from build123d import *

# Parameters (mm, degrees)
F3_D     = 2.5
F3_DEPTH = 16.521
F4_SIZE  = 0.5


with BuildPart() as f1:
    # F0 (on Front) → F1 (revolve)
    with BuildSketch(Plane.XZ):
        Polygon((10, 16), (10, 0), (16.52, 0), (16.52, 2), (13.28, 11), (13.28, 15.774938604), (13.28, 16), align=None)
    revolve(axis=Axis((0, 0, 22.1384353936), (0, 0, 1)))

    # F3 (through all, one way)
    with BuildSketch(Plane.XZ):
        with Locations((0, 13.5)):
            Circle(F3_D / 2)
    extrude(amount=-F3_DEPTH, mode=Mode.SUBTRACT)

    # F4
    f4_edges = [f1.edges().sort_by_distance(p)[0] for p in [
        (-13.28, 0, 16),
        (-10, 0, 16),
        (-10, 0, 0),
        (-16.52, 0, 0),
    ]]
    chamfer(f4_edges, length=F4_SIZE)


solid = f1.part
Geometry: final body of the model. Coordinates: model frame, mm. Round coordinates to 2 decimals unless told otherwise and drop trailing zeros. Write each loop counter-clockwise with the first axis right and the second up, starting at its lowest first coordinate (ties: lowest second). Pieces come first, ordered by that corner, then holes. Notation, with made-up numbers: M 13.25,61 L 39.25,61 A19 ccw 39.25,67 Z; hole C -11,46 d6. An arc over 180 degrees is marked long. Write item = value, one per line.
Item 1: Section query A-A on x = 0. Return loops of the section in (y, z), then the cut area to 3 significant figures.
Findings:
outline = M -16.52,0.5 L -16.02,0 L -10.5,0 L -10,0.5 L -10,15.5 L -10.5,16 L -12.78,16 L -13.28,15.5 L -13.28,11 L -16.52,2 Z; M 10,0.5 L 10.5,0 L 16.02,0 L 16.52,0.5 L 16.52,2 L 13.28,11 L 13.28,12.25 L 10,12.25 Z; M 10,14.75 L 13.28,14.75 L 13.28,15.5 L 12.78,16 L 10.5,16 L 10,15.5 Z
area = 138 mm^2
Item 2: Section query D-D on z = 13.5. Return loops of the section in (x, y), then the cut area to 3 significant figures.
Findings:
outline = M -1.25,9.92 L -1.25,13.22 A13.28 ccw long 1.25,13.22 L 1.25,9.92 A10 cw long Z
area = 232 mm^2
Item 3: Pin query (flat end, axial travel): P1, Ø1.5, axis at x = 11.5, y = 11.5, coming from the -Z side; P2, Ø2, axis at y = -7.5, z = 10.5, coming from the +X side; P3, Ø1.5, axis at x = 4.5, z = 10, coming from the +Y side; P4, Ø2, axis at x = 0, z = 13.5, coming from the +Y side. Return the tip coordinate at first contact, or that it passes through.
Findings:
P1 = 0
P2 = 11.92
P3 = 13.25
P4 = -9.95
Item 4: Pull-direction query (X, two-part tool) for faces 1 (the face through (-10.5, -3.3, 0)), 2 (the face through (-0.16, 11.58, 14.74)), 3 (the face through (7.139, 11.198, 13.282)); classes: pulls with the +X half, pulls with the -X half, needs draft (parallel to the pull), parting line crosses it, or undercut.
Findings:
face_1 = needs draft
face_2 = undercut
face_3 = parting line crosses it
Item 5: Section query C-C on z = 3.5. Return loops of the section in (x, y), then the cut area to 3 significant figures.
Findings:
outline = C 0,0 d31.96; hole C 0,0 d20
area = 488 mm^2
Item 6: Section query B-B on y = 0. Return loops of the section in (x, z), then the cut area to 3 significant figures.
Findings:
outline = M -16.52,0.5 L -16.02,0 L -10.5,0 L -10,0.5 L -10,15.5 L -10.5,16 L -12.78,16 L -13.28,15.5 L -13.28,11 L -16.52,2 Z; M 10,0.5 L 10.5,0 L 16.02,0 L 16.52,0.5 L 16.52,2 L 13.28,11 L 13.28,15.5 L 12.78,16 L 10.5,16 L 10,15.5 Z
area = 146 mm^2
Item 7: Material intervals for line 1 along Z through (x, y) = (0, 10.9); line 2 along Y through (x, z) = (0, 4.25); line 3 along Y through (x, z) = (0.5, 15), sorted ascending. Write a range as [from, to].
Findings:
line_1 = [0, 12.25], [14.75, 16]
line_2 = [-15.71, -10], [10, 15.71]
line_3 = [-13.27, -9.99], [9.99, 13.27]
